from build123d import *

# Parameters (mm, degrees)
SKETCH1_R           = 18.5
SKETCH1_R_2         = 14.5
BOSS_EXTRUDE2_DEPTH = 2
BOSS_EXTRUDE3_START = -2
SKETCH1_4_R         = 18.5
SKETCH1_4_R_2       = 17
BOSS_EXTRUDE3_DEPTH = 2
SKETCH1_5_R         = 15.5
SKETCH1_5_R_2       = 14.5
BOSS_EXTRUDE4_DEPTH = 20
BOSS_EXTRUDE5_START = 20
SKETCH1_6_R         = 15.5
BOSS_EXTRUDE5_DEPTH = 2
SKETCH2_W           = 20
SKETCH2_H           = 20
CUT_EXTRUDE3_DEPTH  = 31
FILLET2_R           = 20
FILLET3_ANGLE       = 240


with BuildPart() as part:
    # Sketch1 → Boss-Extrude2 (new body)
    with BuildSketch(Plane(origin=(0, 0, 0), x_dir=(1, 0, 0), z_dir=(0, 1, 0))):
        with Locations(Location((0, 0, 0), (0, 0, 270))):
            Circle(SKETCH1_R)
        with Locations(Location((0, 0, 0), (0, 0, 270))):
            Circle(SKETCH1_R_2, mode=Mode.SUBTRACT)
    extrude(amount=BOSS_EXTRUDE2_DEPTH)

    # Sketch1<4> → Boss-Extrude3 (add)
    with BuildSketch(Plane(origin=(0, 0, 0), x_dir=(1, 0, 0), z_dir=(0, 1, 0)).offset(BOSS_EXTRUDE3_START)):
        with Locations(Location((0, 0, 0), (0, 0, 270))):
            Circle(SKETCH1_4_R)
        with Locations(Location((0, 0, 0), (0, 0, 270))):
            Circle(SKETCH1_4_R_2, mode=Mode.SUBTRACT)
    extrude(amount=BOSS_EXTRUDE3_DEPTH)

    # Sketch1<5> → Boss-Extrude4 (add)
    with BuildSketch(Plane(origin=(0, 0, 0), x_dir=(1, 0, 0), z_dir=(0, 1, 0))):
        with Locations(Location((0, 0, 0), (0, 0, 270))):
            Circle(SKETCH1_5_R)
        with Locations(Location((0, 0, 0), (0, 0, 270))):
            Circle(SKETCH1_5_R_2, mode=Mode.SUBTRACT)
    extrude(amount=BOSS_EXTRUDE4_DEPTH)

    # Sketch1<6> → Boss-Extrude5 (add)
    with BuildSketch(Plane(origin=(0, 0, 0), x_dir=(1, 0, 0), z_dir=(0, 1, 0)).offset(BOSS_EXTRUDE5_START)):
        with Locations(Location((0, 0, 0), (0, 0, 270))):
            Circle(SKETCH1_6_R)
    extrude(amount=BOSS_EXTRUDE5_DEPTH)

    # Sketch2 → Cut-Extrude3 (cut, symmetric)
    with BuildSketch(Plane(origin=(0, 0, 0), x_dir=(1, 0, 0), z_dir=(0, 1, 0))):
        with Locations((-10, -10)):
            Rectangle(SKETCH2_W, SKETCH2_H)
        Polygon((0, 0), (-20, 11.547005384), (-20, 0), align=None)
    extrude(amount=CUT_EXTRUDE3_DEPTH, both=True, mode=Mode.SUBTRACT)

    # Fillet2
    fillet2_edges = [part.edges().sort_by_distance(p)[0] for p in [
        (0, 21, 0),
    ]]
    fillet(fillet2_edges, radius=FILLET2_R)

    # Fillet3: read off the stored shape, not the designer's step
    # Fillet3 outline → Fillet3 (revolve)
    with BuildSketch(Plane.ZY):
        with BuildLine():
            Line((15.5, 2), (18.5, 2))
            ThreePointArc((18.5, 2), (16.264615938, 7.058428178), (15.5, 12.535653753))
            Line((15.5, 12.535653753), (15.5, 2))
        make_face()
    revolve(axis=Axis((0, 0, 0), (0, 1, 0)), revolution_arc=FILLET3_ANGLE)


solid = part.part
Check sheet for the modelled part. Datum: model origin and axes. Units: mm. A direction names the side the tool comes from. Give positions to 0.01 mm unless a question says otherwise; leave off trailing zeros. Order: outer loops, then holes, each group sorted by start corner. A loop starts at its lowest first (then second) coordinate and runs counter-clockwise, first axis right, second up. Notation, with made-up numbers: M 49.5,61.5 L 59.5,61.5 A9 ccw 59.5,65.5 Z; hole C 25.25,64 d5. An arc over 180 degrees is marked long. Answer as CSV lines item,"result". Start each with the question number.
Item 1: Tool access check on faces 5 (the face through (0, 8.3, 15.5)), 6 (the face through (12, 0, -9)), 7 (the face through (13.645, 17.202, -7.353)). Record the directions out of +Z, -Z, +X, -X, +Y, -Y that give a thin tool (end or side, any length) a straight path to the whole face; none if there is none.
Item 2: Thickness scan on line 1 (X direction, y = -0.55, z = 0); line 2 (Y direction, x = -7.5, z = -7); line 3 (X direction, y = 13.5, z = 0). Record the ranges inside material, lowest first. Write a range as [from, to].
Item 3: Cross-section at C-C on y = 13.75. Enter the section's corners in (x, z), plus the area to 3 significant figures.
Item 4: Cross-section at B-B on z = 0. Enter the section's corners in (x, y).
Item 5: Gauge pin test, flat ends, axial feed: P1, Ø12, axis at x = -10, y = 10.5, coming from the -Z side; P2, Ø2, axis at x = 9, y = 3, coming from the -Z side; P3, Ø3, axis at y = 3.5, z = -4, coming from the +X side; P4, Ø1.5, axis at x = 15, z = 6.5, coming from the -Y side. Record the tip position at first contact, or that the pin passes through.
Item 6: Mould release check, pull along X, two halves, no side actions. Record for faces 1 (the face through (4, 20, -3)), 2 (the face through (16.286, -0.028, -8.776)), 3 (the face through (4, 22, -4)), 4 (the face through (12.765, 9.86, -6.879)): +X half, -X half, draft (parallel to the pull), parting line (faces both ways), or undercut.
Item 7: Cross-section at A-A on y = 8. Enter the section's corners in (x, z).
Established:
1,face 5,"+Z, -X, +Y, -Y"
1,face 6,"-Y"
1,face 7,"+Y"
2,line 1,"x = [17, 18.5]"
2,line 2,"y = [20, 22]"
2,line 3,"x = [14.5, 15.5]"
3,outline,"M -13.42,-7.75 A15.5 ccw long 0,15.5 L 0,14.5 A14.5 cw long -12.56,-7.25 Z"
3,area,"62.8 mm^2"
4,outline,"M -3.67,20 L 14.5,20 L 14.5,0 L 17,0 L 17,-2 L 18.5,-2 L 18.5,2 A20 cw 15.5,12.54 L 15.5,22 L -3.67,22 Z"
5,P1,"stops at z = -15.48"
5,P2,"stops at z = -16.35"
5,P3,"stops at x = 18.11"
5,P4,"stops at y = -2"
6,face 1,"undercut"
6,face 2,"parting line"
6,face 3,"draft"
6,face 4,"undercut"
7,outline,"M -13.87,-8.01 A16.02 ccw long 0,16.02 L 0,14.5 A14.5 cw long -12.56,-7.25 Z"
